Here's the drawing with two shaded views (mm, measured from the low corner). I have some questions. Round coordinates to 2 decimals unless told otherwise and drop trailing zeros. Order: outer loops, then holes, each group sorted by start corner. A loop starts at its lowest first (then second) coordinate and runs counter-clockwise, first axis right, second up. Notation, with made-up numbers: (8.5, -31.5) -> (65.5, -31.5) arc R21 cw to (65.5, 6.5) -> close; hole circle Ø4 at (73, 71). An arc over 180 degrees is marked (long way). Answer in a Markdown table with one row per item.
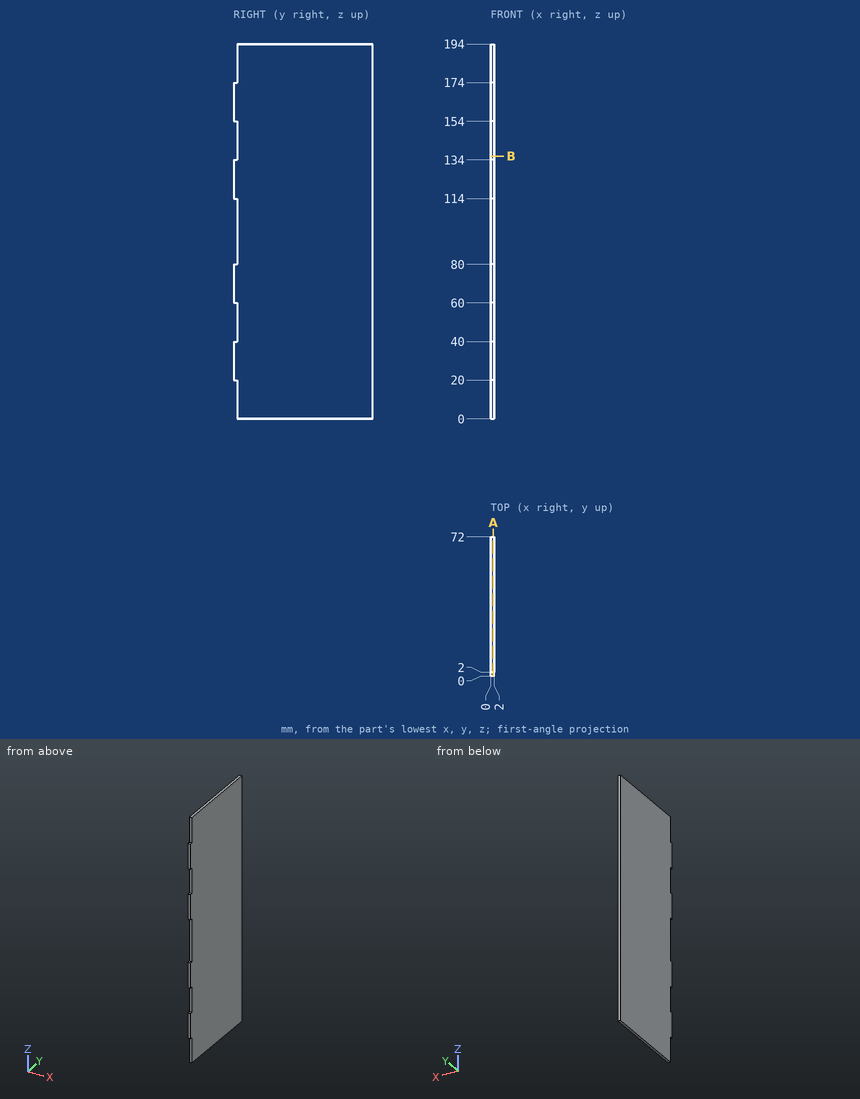
1. For pin 1 Ø1 at (x, z) = (1, 12) entering from -Y; pin 2 Ø1 at (x, y) = (1, 0.5) entering from -Z; pin 3 Ø1 at (x, y) = (0.5, 1) entering from +Z, each with a flat end and sliding along its axis, tell me the tip position at first contact or that it passes through.
Numbers:
| item | result |
|---|---|
| pin 1 | stops at y = 2 |
| pin 2 | stops at z = 20 |
| pin 3 | stops at z = 174 |
2. Suppose I cut it at A-A on x = 1.45. Write out the boundary of the cut face in (y, z), then the cut area to 3 significant figures.
Numbers:
| item | result |
|---|---|
| outline | (0, 20) -> (2, 20) -> (2, 0) -> (72, 0) -> (72, 194) -> (2, 194) -> (2, 174) -> (0, 174) -> (0, 154) -> (2, 154) -> (2, 134) -> (0, 134) -> (0, 114) -> (2, 114) -> (2, 80) -> (0, 80) -> (0, 60) -> (2, 60) -> (2, 40) -> (0, 40) -> close |
| area | 13,700 mm2 |
3. Suppose I cut it at B-B on z = 136. Write out the boundary of the cut face in (x, y).
Numbers:
| item | result |
|---|---|
| outline | (0, 2) -> (2, 2) -> (2, 72) -> (0, 72) -> close |
4. Please list where this line runs through material, in increasing order: line 1 along Y through (x, z) = (0.65, 148.5).
Numbers:
| item | result |
|---|---|
| line 1 | y = 2 to 72 |
